Build history of the part. All positions in model axes, mm. Face numbers are marked on the shaded views. A direction names the side the tool comes from. Coordinates: 2 decimals unless noted, no trailing zeros. Order: outer loops, then holes, each group sorted by start corner. A loop starts at its lowest first (then second) coordinate and runs counter-clockwise, first axis right, second up. Notation, with made-up numbers: (38.5, 14.5) -> (87.5, 14.5) arc R18 ccw to (87.5, 40.5) -> close; hole circle Ø6 at (51.5, 84). An arc over 180 degrees is marked (long way). Write each question's results on one line, items separated by ' | '.
from build123d import *

# Parameters (mm, degrees)
F1_DEPTH = 100
F2_SIZE  = 59.99999


# Not quite as in the source:
# - a fillet or chamfer is up to 0.001 mm smaller than in the source, because OpenCascade refuses the exact size


with BuildPart() as f1:
    # F0 (on Right) → F1 (new body)
    with BuildSketch(Plane.YZ):
        Polygon((-60, 0), (0, 0), (0, 60), (-20, 60), (-20, 40), (-40, 40), (-40, 20), (-60, 20), align=None)
    extrude(amount=F1_DEPTH)

    # F2 (size 60 in the source; OpenCascade refuses exactly that, so slightly less here)
    f2_edges = [f1.edges().sort_by_distance(p)[0] for p in [
        (100, -10, 60),
    ]]
    chamfer(f2_edges, length=F2_SIZE)


solid = f1.part
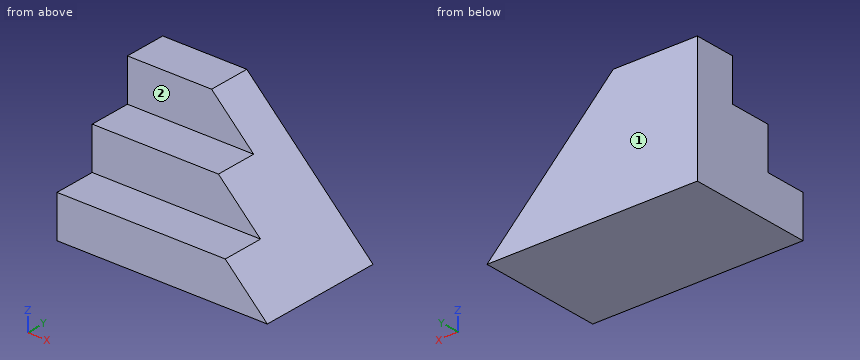
Item 1: Pin check, flat tips, straight feed: pin 1 (10 mm diameter, centred on y = -24, z = 32.5, fed in from +X); pin 2 (16 mm diameter, centred on x = 28, z = 45.5, fed in from -Y); pin 3 (2 mm diameter, centred on y = -15.5, z = 30, fed in from +X). Stop position of each tip, or through.
Answer:
pin 1: stops at x = 72.5 | pin 2: stops at y = -40 | pin 3: stops at x = 71
Item 2: Slice it at C-C, the plane z = 10.5. List the corners of the cut face in (x, y), and give its area (3 significant figures).
Answer:
outline: (0, -60) -> (89.5, -60) -> (89.5, 0) -> (0, 0) -> close | area: 5,370 mm^2
Item 3: Tool access for the marked faces 1 and 2: list every direction of +Z, -Z, +X, -X, +Y, -Y with a clear straight run to the whole face (end or side of a thin tool).
Answer:
face 1: +Z, -Z, +X, -X, +Y | face 2: +Z, +X, -X, -Y
Item 4: Drill centre lines: line 1 (Y direction, x = 12, z = 31); line 2 (Z direction, x = 11, y = -34.5); line 3 (Y direction, x = 7, z = 46.5). Where is each one in solid material? Low to high. Write a range as from..to.
Answer:
line 1: y = -40..0 | line 2: z = 0..40 | line 3: y = -20..0
Item 5: Slice it at A-A, the plane x = 20. List the corners of the cut face in (y, z), and give its area (3 significant figures).
Answer:
outline: (-60, 0) -> (0, 0) -> (0, 60) -> (-20, 60) -> (-20, 40) -> (-40, 40) -> (-40, 20) -> (-60, 20) -> close | area: 2,400 mm^2
